```python
from build123d import *

# Parameters (mm, degrees)
BOSS_EXTRUDE1_DEPTH = 71.12
CUT_EXTRUDE1_REACH  = 5.175
SKETCH2_R           = 2.0193
SKETCH3_R           = 2.5527
CUT_EXTRUDE2_DEPTH  = 51.8


with BuildPart() as part:
    # Sketch1 → Boss-Extrude1 (new body)
    with BuildSketch(Plane.XY):
        Polygon((47.625, 3.175), (47.625, 25.4), (50.8, 25.4), (50.8, 0), (0, 0), (0, 25.4), (3.175, 25.4), (3.175, 3.175), align=None)
    extrude(amount=BOSS_EXTRUDE1_DEPTH)

    # Sketch2 → Cut-Extrude1 (cut, up to next)
    with BuildSketch(Plane(origin=(0, 3.175, 0), x_dir=(1, 0, 0), z_dir=(0, 1, 0)), mode=Mode.PRIVATE) as cut_extrude1_sk1:
        with Locations((38.1, -4.4975)):
            Circle(SKETCH2_R)
    cut_extrude1_tool1 = extrude(cut_extrude1_sk1.sketch, amount=-CUT_EXTRUDE1_REACH, mode=Mode.PRIVATE) & part.part
    add(cut_extrude1_tool1.solids().sort_by_distance((38.1, 3.175, 4.4975))[0], mode=Mode.SUBTRACT)
    # Sketch2 → Cut-Extrude1 (cut, up to next)
    with BuildSketch(Plane(origin=(0, 3.175, 0), x_dir=(1, 0, 0), z_dir=(0, 1, 0)), mode=Mode.PRIVATE) as cut_extrude1_sk2:
        with Locations((38.1, -61.6475)):
            Circle(SKETCH2_R)
    cut_extrude1_tool2 = extrude(cut_extrude1_sk2.sketch, amount=-CUT_EXTRUDE1_REACH, mode=Mode.PRIVATE) & part.part
    add(cut_extrude1_tool2.solids().sort_by_distance((38.1, 3.175, 61.6475))[0], mode=Mode.SUBTRACT)
    # Sketch2 → Cut-Extrude1 (cut, up to next)
    with BuildSketch(Plane(origin=(0, 3.175, 0), x_dir=(1, 0, 0), z_dir=(0, 1, 0)), mode=Mode.PRIVATE) as cut_extrude1_sk3:
        with Locations((12.7, -4.4975)):
            Circle(SKETCH2_R)
    cut_extrude1_tool3 = extrude(cut_extrude1_sk3.sketch, amount=-CUT_EXTRUDE1_REACH, mode=Mode.PRIVATE) & part.part
    add(cut_extrude1_tool3.solids().sort_by_distance((12.7, 3.175, 4.4975))[0], mode=Mode.SUBTRACT)
    # Sketch2 → Cut-Extrude1 (cut, up to next)
    with BuildSketch(Plane(origin=(0, 3.175, 0), x_dir=(1, 0, 0), z_dir=(0, 1, 0)), mode=Mode.PRIVATE) as cut_extrude1_sk4:
        with Locations((12.7, -61.6475)):
            Circle(SKETCH2_R)
    cut_extrude1_tool4 = extrude(cut_extrude1_sk4.sketch, amount=-CUT_EXTRUDE1_REACH, mode=Mode.PRIVATE) & part.part
    add(cut_extrude1_tool4.solids().sort_by_distance((12.7, 3.175, 61.6475))[0], mode=Mode.SUBTRACT)

    # Sketch3 → Cut-Extrude2 (cut, through all)
    with BuildSketch(Plane(origin=(50.8, 0, 0), x_dir=(0, 0, -1), z_dir=(1, 0, 0))):
        with Locations((-6.35, 15.875)):
            Circle(SKETCH3_R)
        with Locations((-64.77, 15.875)):
            Circle(SKETCH3_R)
    extrude(amount=-CUT_EXTRUDE2_DEPTH, mode=Mode.SUBTRACT)


solid = part.part
```
CAD build for the part. Positions are in the model's coordinates, mm. A direction names the side the tool comes from. Round coordinates to 2 decimals unless told otherwise and drop trailing zeros. Loops run counter-clockwise (first coordinate to the right, second up) from the corner with the lowest first, then second, coordinate; pieces in that order, holes last. Notation, with made-up numbers: (66, 28.5) - (82, 28.5) arc R25 ccw to (82, 58.5) - close; hole circle Ø3 at (-31.75, 16). An arc over 180 degrees is marked (long way). Return JSON: item names as keys, results as strings. Group by question number.
Q1. Tool access for faces 1 (the face through (49, 25.4, 35)), 2 (the face through (47.625, 14, 35)): list every direction of +Z, -Z, +X, -X, +Y, -Y with a clear straight run to the whole face (end or side of a thin tool).
Q2. Drill centre lines: line 1 along Z through (x, y) = (12.7, 1.6); line 2 along X through (y, z) = (13.5, 14) (3 decimals); line 3 along Y through (x, z) = (1.85, 64.77). Where is each one in solid material? Low to high. Write a range as [from, to].
Q3. Band-saw the part on B-B on y = 5. Give the cut face in (x, z) (3 decimals), plus the area to 3 significant figures.
Q4. Band-saw the part on C-C on z = 64.77. Give the cut face in (x, y) (3 decimals), plus the area to 3 significant figures.
Q5. Band-saw the part on D-D on z = 43. Give the cut face in (x, y) (3 decimals).
Q6. Flat gauge pin, fed straight in: pin 1 Ø4 at (x, z) = (24.5, 44) entering from +Y (3 decimals). Where does the tip first touch, or does it go through?
Q7. Two-plate mould, pull along Y, no slides. Class faces 3 (the face through (1.61, 15.99, 67.32)), 4 (the face through (2, 25.4, 35)), 5 (the face through (24, 2, 71.12)): +Y half, -Y half, draft (parallel to the pull), parting line (faces both ways), or undercut.
Q8. Band-saw the part on A-A on x = 38.1. Give the cut face in (y, z) (3 decimals), plus the area to 3 significant figures.
Solutions:
{
 "1": {"face 1": "+Z, -Z, +X, -X, +Y", "face 2": "+Z, -Z, +Y"},
 "2": {"line 1": "z = [0, 2.48], [6.52, 59.63], [63.67, 71.12]", "line 2": "x = [0, 3.175], [47.625, 50.8]", "line 3": "y = [0, 13.32], [18.43, 25.4]"},
 "3": {"outline": "(0, 0) - (3.175, 0) - (3.175, 71.12) - (0, 71.12) - close; (47.625, 0) - (50.8, 0) - (50.8, 71.12) - (47.625, 71.12) - close", "area": "452 mm^2"},
 "4": {"outline": "(0, 0) - (50.8, 0) - (50.8, 13.322) - (47.625, 13.322) - (47.625, 3.175) - (3.175, 3.175) - (3.175, 13.322) - (0, 13.322) - close; (0, 18.428) - (3.175, 18.428) - (3.175, 25.4) - (0, 25.4) - close; (47.625, 18.428) - (50.8, 18.428) - (50.8, 25.4) - (47.625, 25.4) - close", "area": "270 mm^2"},
 "5": {"outline": "(0, 0) - (50.8, 0) - (50.8, 25.4) - (47.625, 25.4) - (47.625, 3.175) - (3.175, 3.175) - (3.175, 25.4) - (0, 25.4) - close"},
 "6": {"pin 1": "stops at y = 3.175"},
 "7": {"face 3": "undercut", "face 4": "+Y half", "face 5": "draft"},
 "8": {"outline": "(0, 0) - (3.175, 0) - (3.175, 2.478) - (0, 2.478) - close; (0, 6.517) - (3.175, 6.517) - (3.175, 59.628) - (0, 59.628) - close; (0, 63.667) - (3.175, 63.667) - (3.175, 71.12) - (0, 71.12) - close", "area": "200 mm^2"}
}
